Geometry: see drawing. Coordinates: mm, zero at the bounding-box minimum. A direction names the side the tool comes from. Round coordinates to 2 decimals unless told otherwise and drop trailing zeros. Write each loop counter-clockwise with the first axis right and the second up, starting at its lowest first coordinate (ties: lowest second). Pieces come first, ordered by that corner, then holes. Notation, with made-up numbers: (-39, -25.5) -> (14, -25.5) arc R18 ccw to (14, -7.5) -> close; hole circle Ø3 at (89, 74). An arc over 180 degrees is marked (long way). Write item = value, one per line. Start each with the question number.
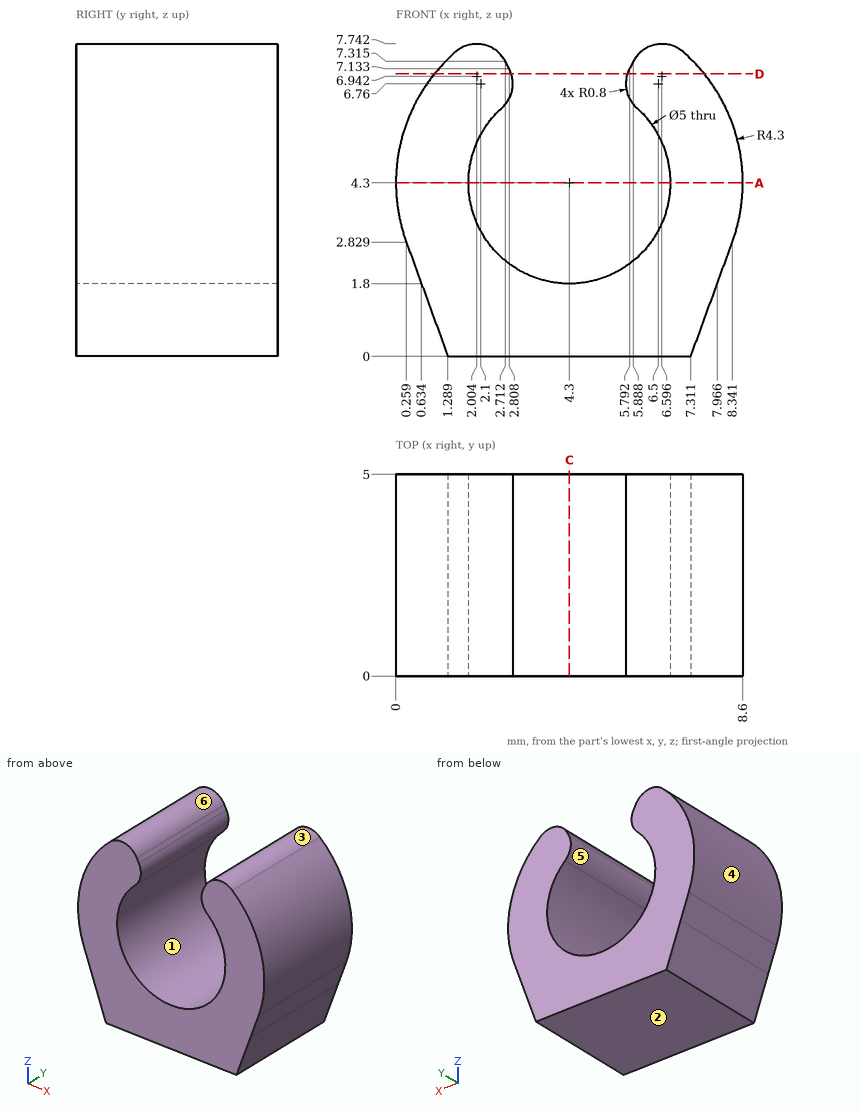
1. Line query: line 1 along X through (y, z) = (1.45, 4.3); line 2 along Z through (x, y) = (4.3, 2); line 3 along X through (y, z) = (1.1, 3.25). Output: solid intervals per line, ascending.
2. Section A-A (z = 4.3). Output: boundary loops of the cut face in (x, y).
3. Pin query (flat end, axial travel): P1, Ø3, axis at y = 3.5, z = 1, coming from the +X side; P2, Ø2, axis at x = 4, y = 2.5, coming from the +Z side (1 decimal); P3, Ø3, axis at y = 3.5, z = 7, coming from the -X side. Return the tip coordinate at first contact, or that it passes through.
4. Reachability of the marked faces 5 and 6 from +Z, -Z, +X, -X, +Y, -Y: full face, straight path, thin tool, end or side. Return the list, or none.
5. Mould query, pull axis X, two halves, no side actions, for the marked faces 1, 2, 3 and 4. Classes: pulls with the +X half, pulls with the -X half, needs draft (parallel to the pull), parting line crosses it, or undercut.
6. Section C-C (x = 4.3). Output: boundary loops of the cut face in (y, z).
7. Section D-D (z = 7). Output: boundary loops of the cut face in (x, y).
Check sheet entries:
q1.line_1 = 0 to 1.8, 6.8 to 8.6
q1.line_2 = 0 to 1.8
q1.line_3 = 0.13 to 2.03, 6.57 to 8.47
q2.outline = (0, 0) -> (1.8, 0) -> (1.8, 5) -> (0, 5) -> close; (6.8, 0) -> (8.6, 0) -> (8.6, 5) -> (6.8, 5) -> close
q3.P1 = 8.22
q3.P2 = 2.2
q3.P3 = 0.17
q4.face_5 = +Y, -Y
q4.face_6 = +Z, +Y, -Y
q5.face_1 = undercut
q5.face_2 = needs draft
q5.face_3 = undercut
q5.face_4 = pulls with the -X half
q6.outline = (0, 0) -> (5, 0) -> (5, 1.8) -> (0, 1.8) -> close
q7.outline = (0.95, 0) -> (2.86, 0) -> (2.86, 5) -> (0.95, 5) -> close; (5.74, 0) -> (7.65, 0) -> (7.65, 5) -> (5.74, 5) -> close
